from build123d import *

# Parameters (mm, degrees)
PAD003_DEPTH    = 60
SKETCH022_R     = 4.05
POCKET018_DEPTH = 332.001
SKETCH023_R     = 8.65
POCKET019_DEPTH = 4
SKETCH024_R     = 4.05
POCKET020_DEPTH = 332.001
FILLET006_R     = 1
FILLET007_R     = 1


with BuildPart() as part:
    # Sketch021 → Pad003 (new body)
    with BuildSketch(Plane.XZ.offset(25)):
        Polygon((332, 31), (332, 50.05), (329, 50.05), (322, 40.05), (322, 21.95), (329, 11.95), (332, 11.95), align=None)
    extrude(amount=PAD003_DEPTH)

    # Sketch022 → Pocket018 (cut, through all)
    with BuildSketch(Plane.YZ):
        with Locations((-75, 31)):
            Circle(SKETCH022_R)
        with Locations((-35, 31)):
            Circle(SKETCH022_R)
    extrude(amount=POCKET018_DEPTH, mode=Mode.SUBTRACT)

    # Sketch023 → Pocket019 (cut)
    with BuildSketch(Plane.YZ.offset(322)):
        with Locations((-75, 31)):
            Circle(SKETCH023_R)
        with Locations((-35, 31)):
            Circle(SKETCH023_R)
    extrude(amount=POCKET019_DEPTH, mode=Mode.SUBTRACT)

    # Sketch024 → Pocket020 (cut, through all)
    with BuildSketch(Plane.YZ):
        with Locations((-55, 31)):
            Circle(SKETCH024_R)
    extrude(amount=POCKET020_DEPTH, mode=Mode.SUBTRACT)

    # Fillet006
    fillet006_edges = [part.edges().sort_by_distance(p)[0] for p in [
        (329, -55, 11.95),
        (322, -55, 21.95),
        (322, -55, 40.05),
        (329, -55, 50.05),
    ]]
    fillet(fillet006_edges, radius=FILLET006_R)

    # Fillet007
    fillet007_edges = [part.edges().sort_by_distance(p)[0] for p in [
        (325.441096, -25, 44.965851),
        (322, -25, 31),
        (325.441096, -25, 17.034149),
        (325.441096, -85, 17.034149),
        (322, -85, 31),
        (325.441096, -85, 44.965851),
    ]]
    fillet(fillet007_edges, radius=FILLET007_R)


solid = part.part
Work out the finished part from the listing and answer in its coordinate system (mm). A direction names the side the tool comes from. Coordinates: 2 decimals unless noted, no trailing zeros. Loops run counter-clockwise (first coordinate to the right, second up) from the corner with the lowest first, then second, coordinate; pieces in that order, holes last. Notation, with made-up numbers: M 84,70.25 L 95,70.25 A15 ccw 95,90.25 Z; hole C 50,69 d5. An arc over 180 degrees is marked long. Answer in a Markdown table with one row per item. Add a question column.
1. Find section A-A, the plane y = -55. Write down the section's boundary in (x, z).
2. Find section D-D, the plane y = -75. Write down the section's boundary in (x, z), then the cut area to 3 significant figures.
3. Consider L1, parallel to Y at x = 328.5, z = 31; L2, parallel to Z at x = 329.55, y = -75; L3, parallel to Y at x = 326.25, z = 17.5. Determine where each line is inside the solid, lowest interval first.
4. A tool of negligible diameter and unlimited length cuts with its end or side. For faces 1 (the flat face through (326, -71, 29)), 2 (the cylindrical face through (325.64, -84.71, 44.73)), from which of +Z, -Z, +X, -X, +Y, -Y can it reach the whole face along a straight path? Write none if from no direction.
5. Find section C-C, the plane x = 331. Write down the section's boundary in (y, z).
6. The mould has two halves that part along Z. Classify faces 3 (the flat face through (322, -55, 37)), 4 (the cylindrical face through (323.972, -41.375, 36.846)), 5 (the flat face through (331, -55, 50.05)): pulls with the +Z half, pulls with the -Z half, needs draft (parallel to the pull), parting line crosses it, or undercut.
7. Find section B-B, the plane z = 31. Write down the section's boundary in (x, y), then the cut area to 3 significant figures.
8. Flat-ended cylindrical pins translate along their axes: P1, Ø9.5, axis at y = -35, z = 31, coming from the -X side; P2, Ø1, axis at x = 323, y = -45, coming from the +Z side; P3, Ø1.5, axis at y = -44, z = 43, coming from the -X side. Find the tip coordinate at first contact, or state that the pin passes through.
Reported:
| question | item | result |
|---|---|---|
| 1 | outline | M 322,22.27 A1 ccw 322.18,21.69 L 328.7,12.38 A1 ccw 329.52,11.95 L 332,11.95 L 332,26.95 L 322,26.95 Z; M 322,35.05 L 332,35.05 L 332,50.05 L 329.52,50.05 A1 ccw 328.7,49.62 L 322.18,40.31 A1 ccw 322,39.73 Z |
| 2 | outline | M 322,22.27 A1 ccw 322.18,21.69 L 328.7,12.38 A1 ccw 329.52,11.95 L 332,11.95 L 332,26.95 L 326,26.95 L 326,22.35 L 322,22.35 Z; M 322,39.65 L 326,39.65 L 326,35.05 L 332,35.05 L 332,50.05 L 329.52,50.05 A1 ccw 328.7,49.62 L 322.18,40.31 A1 ccw 322,39.73 Z |
| 2 | area | 193 mm^2 |
| 3 | L1 | y = -85 to -79.05, -70.95 to -59.05, -50.95 to -39.05, -30.95 to -25 |
| 3 | L2 | z = 11.95 to 26.95, 35.05 to 50.05 |
| 3 | L3 | y = -85 to -25 |
| 4 | face 1 | -X |
| 4 | face 2 | +Z, -X, -Y |
| 5 | outline | M -85,12.95 A1 ccw -84,11.95 L -26,11.95 A1 ccw -25,12.95 L -25,49.05 A1 ccw -26,50.05 L -84,50.05 A1 ccw -85,49.05 Z; hole C -75,31 d8.1; hole C -55,31 d8.1; hole C -35,31 d8.1 |
| 6 | face 3 | needs draft |
| 6 | face 4 | undercut |
| 6 | face 5 | pulls with the +Z half |
| 7 | outline | M 322,-84 A1 ccw 323,-85 L 332,-85 L 332,-79.05 L 326,-79.05 L 326,-83.65 L 322,-83.65 Z; M 322,-66.35 L 326,-66.35 L 326,-70.95 L 332,-70.95 L 332,-59.05 L 322,-59.05 Z; M 322,-50.95 L 332,-50.95 L 332,-39.05 L 326,-39.05 L 326,-43.65 L 322,-43.65 Z; M 322,-26.35 L 326,-26.35 L 326,-30.95 L 332,-30.95 L 332,-25 L 323,-25 A1 ccw 322,-26 Z |
| 7 | area | 283 mm^2 |
| 8 | P1 | stops at x = 326 |
| 8 | P2 | stops at z = 42.19 |
| 8 | P3 | stops at x = 323.54 |
